CAD build for the part. Positions are in the model's coordinates, mm. A direction names the side the tool comes from. Give positions to 0.01 mm unless a question says otherwise; leave off trailing zeros. Order: outer loops, then holes, each group sorted by start corner. A loop starts at its lowest first (then second) coordinate and runs counter-clockwise, first axis right, second up. Notation, with made-up numbers: (63, 33) -> (99, 33) arc R19 ccw to (99, 52) -> close; hole circle Ø2 at (2.25, -12.5). An arc over 180 degrees is marked (long way). Use one line per item in the form item = value. Start each with the question number.
1) Probe line 1 (X direction, y = -2.25, z = 1.75); line 2 (Y direction, x = -11.5, z = -2); line 3 (X direction, y = 2.25, z = -1.5). List the from-to ranges inside material, lowest first.
2) Mould opens along Y. For faces 1 (the face through (3.52, -2.79, 2.08)), 2 (the face through (0, 9.03, 0)), 3 (the face through (-12, -0.758, -2)), 4 (the face through (12.766, -6, -2)) say: pulls with the +Y half, pulls with the -Y half, needs draft (parallel to the pull), parting line crosses it, or undercut.
3) Cut at A-A, the plane z = 2.75. Give the cut face in (x, y).
4) Tool access for faces 5 (the face through (-6.388, 0, 2)), 6 (the face through (-12, -3.95, -2)), 7 (the face through (14, -5.465, -2)): list every direction of +Z, -Z, +X, -X, +Y, -Y with a clear straight run to the whole face (end or side of a thin tool).
5) Cut at D-D, the plane x = -12.5. Give the cut face in (y, z), and give its area (3 significant figures).
6) Drop flat-ended pins along their axis: P1, Ø0.9, axis at x = -13, z = -2, coming from the +Y side; P2, Ø8, axis at x = -3, y = 0, coming from the +Z side; P3, Ø1.5, axis at y = 1.5, z = -0.5, coming from the +X side; P4, Ø3, axis at x = -4.5, z = 1.5, coming from the -Y side. Give the stop position or say it passes through.
7) Cut at B-B, the plane z = -1.75. Give the cut face in (x, y).
8) Cut at C-C, the plane y = -6.5. Give the cut face in (x, z).
from build123d import *

# Parameters (mm, degrees)
F0_W     = 43.2562
F0_H     = 18.0594
F1_DEPTH = 0.8255
F2_W     = 9.271
F2_H     = 7.6454
F3_DEPTH = 3.81
F4_W     = 3.7084
F4_H     = 6.1214
F5_DEPTH = 2.54
F6_W     = 10.16
F6_H     = 5.207
F6_W_2   = 3.4798
F6_H_2   = 1.6764
F6_W_3   = 3.5052
F6_H_3   = 8.043443
F7_DEPTH = 1.778


with BuildPart() as f1:
    # F0 (on Top) → F1 (new body, symmetric)
    with BuildSketch(Plane.XY):
        Rectangle(F0_W, F0_H)
    extrude(amount=F1_DEPTH, both=True)

    # F2 (on face) → F3 (join)
    with BuildSketch(Plane.XY.offset(0.8255)):
        with Locations((18.669, 0)):
            Rectangle(F2_W, F2_H)
    extrude(amount=F3_DEPTH)

    # F4 (on face) → F5 (join)
    with BuildSketch(Plane.XY.offset(0.8255)):
        with Locations((-4.5339, 0)):
            Rectangle(F4_W, F4_H)
        Polygon((12.045661, 0), (6.3881, 5.657561), (0.730539, 0), (6.3881, -5.657561), align=None)
    extrude(amount=F5_DEPTH)

    # F6 (on face) → F7 (join)
    with BuildSketch(Plane(origin=(0, 0, -0.8255), x_dir=(1, 0, 0), z_dir=(0, 0, -1))):
        with Locations((8.8011, 0)):
            Rectangle(F6_W, F6_H)
        with Locations((14.50628, 6.303569)):
            Rectangle(F6_W_2, F6_H_2)
        with Locations((-12.138053, -3.263815)):
            Rectangle(F6_W_3, F6_H_3)
        with Locations((-11.713614, 3.1115)):
            Rectangle(F6_W_2, F6_H_2)
    extrude(amount=F7_DEPTH)


solid = f1.part
Result:
q1.line_1 = -6.39 to -2.68, 2.98 to 9.8, 14.03 to 23.3
q1.line_2 = -3.95 to -2.27, -0.76 to 7.29
q1.line_3 = -13.89 to -10.39, 3.72 to 13.88
q2.face_1 = pulls with the -Y half
q2.face_2 = pulls with the +Y half
q2.face_3 = undercut
q2.face_4 = needs draft
q3.outline = (-6.39, -3.06) -> (-2.68, -3.06) -> (-2.68, 3.06) -> (-6.39, 3.06) -> close; (0.73, 0) -> (6.39, -5.66) -> (12.05, 0) -> (6.39, 5.66) -> close; (14.03, -3.82) -> (23.3, -3.82) -> (23.3, 3.82) -> (14.03, 3.82) -> close
q4.face_5 = +Z, -X, +Y, -Y
q4.face_6 = -Z, +X, -X, -Y
q4.face_7 = -Z, +X, -X
q5.outline = (-9.03, -0.83) -> (-3.95, -0.83) -> (-3.95, -2.6) -> (-2.27, -2.6) -> (-2.27, -0.83) -> (-0.76, -0.83) -> (-0.76, -2.6) -> (7.29, -2.6) -> (7.29, -0.83) -> (9.03, -0.83) -> (9.03, 0.83) -> (-9.03, 0.83) -> close
q5.area = 47.1 mm²
q6.P1 = 7.29
q6.P2 = 3.37
q6.P3 = 21.63
q6.P4 = -9.03
q7.outline = (-13.89, -0.76) -> (-10.39, -0.76) -> (-10.39, 7.29) -> (-13.89, 7.29) -> close; (-13.45, -3.95) -> (-9.97, -3.95) -> (-9.97, -2.27) -> (-13.45, -2.27) -> close; (3.72, -2.6) -> (13.88, -2.6) -> (13.88, 2.6) -> (3.72, 2.6) -> close; (12.77, -7.14) -> (16.25, -7.14) -> (16.25, -5.47) -> (12.77, -5.47) -> close
q8.outline = (-21.63, -0.83) -> (12.77, -0.83) -> (12.77, -2.6) -> (16.25, -2.6) -> (16.25, -0.83) -> (21.63, -0.83) -> (21.63, 0.83) -> (-21.63, 0.83) -> close
